from build123d import *

# Parameters (mm, degrees)
BOSS_EXTRUDE1_DEPTH = 2
SKETCH2_R           = 1.5
CUT_EXTRUDE1_DEPTH  = 31.987900865
SKETCH3_R           = 2.25
SKETCH3_R_2         = 1.5
BOSS_EXTRUDE2_DEPTH = 0.5
FILLET1_R           = 5


with BuildPart() as part:
    # Sketch1 → Boss-Extrude1 (new body)
    with BuildSketch(Plane(origin=(0, 0, 0), x_dir=(1, 0, 0), z_dir=(0, 1, 0))):
        with BuildLine():
            Line((7.5, 22.5), (7.5, -22.5))
            ThreePointArc((7.5, -22.5), (0, -30), (-7.5, -22.5))
            Line((-7.5, -22.5), (-7.5, 22.5))
            ThreePointArc((-7.5, 22.5), (0, 30), (7.5, 22.5))
        make_face()
    extrude(amount=BOSS_EXTRUDE1_DEPTH)

    # Sketch2 → Cut-Extrude1 (cut, through all)
    with BuildSketch(Plane(origin=(0, 2, 0), x_dir=(1, 0, 0), z_dir=(0, 1, 0))):
        with Locations(Location((0, 22.5, 0), (0, 0, 270))):
            Circle(SKETCH2_R)
        with Locations(Location((0, -22.5, 0), (0, 0, 270))):
            Circle(SKETCH2_R)
    extrude(amount=-CUT_EXTRUDE1_DEPTH, mode=Mode.SUBTRACT)

    # Sketch3 → Boss-Extrude2 (add)
    # profile 1 of 2: a face of its own
    with BuildSketch(Plane.XZ):
        with Locations(Location((0, 22.5, 0), (0, 0, 90))):
            Circle(SKETCH3_R)
        with Locations(Location((0, 22.5, 0), (0, 0, 90))):
            Circle(SKETCH3_R_2, mode=Mode.SUBTRACT)
    # profile 2 of 2: a face of its own
    with BuildSketch(Plane.XZ):
        with Locations(Location((0, -22.5, 0), (0, 0, 90))):
            Circle(SKETCH3_R)
        with Locations(Location((0, -22.5, 0), (0, 0, 90))):
            Circle(SKETCH3_R_2, mode=Mode.SUBTRACT)
    extrude(amount=BOSS_EXTRUDE2_DEPTH)

    # Fillet1
    # the kernel refuses this fillet: 5 mm, written as the material it adds along each edge
    with BuildSketch(Plane(origin=(0, 0, 22.5), x_dir=(0, 0, 1), z_dir=(1, 0, 0))) as fillet1_piece_1:
        with BuildLine():
            CenterArc((4.429449472, 5), FILLET1_R, 244.158067237, 25.841932763)
            Line((2.25, 0.5), (2.206411011, 0.41))
            ThreePointArc((2.206411011, 0.41), (2.15, 0.25), (2.15, 0))
            Line((2.15, 0), (2.25, -0.1))
            Line((2.25, -0.1), (4.429449472, -0.1))
            Line((4.429449472, -0.1), (4.429449472, 0))
        make_face()
    revolve(axis=Axis((0, 0, 22.5), (0, -1, 0)))
    with BuildSketch(Plane(origin=(0, 0, -22.5), x_dir=(0, 0, 1), z_dir=(1, 0, 0))) as fillet1_piece_2:
        with BuildLine():
            CenterArc((4.429449472, 5), FILLET1_R, 244.158067237, 25.841932763)
            Line((2.25, 0.5), (2.206411011, 0.41))
            ThreePointArc((2.206411011, 0.41), (2.15, 0.25), (2.15, 0))
            Line((2.15, 0), (2.25, -0.1))
            Line((2.25, -0.1), (4.429449472, -0.1))
            Line((4.429449472, -0.1), (4.429449472, 0))
        make_face()
    revolve(axis=Axis((0, 0, -22.5), (0, -1, 0)))


solid = part.part
Model file for the job. Use its own axes, mm. Coordinates: 2 decimals unless noted, no trailing zeros. Order: outer loops, then holes, each group sorted by start corner. A loop starts at its lowest first (then second) coordinate and runs counter-clockwise, first axis right, second up. Notation, with made-up numbers: (63, 8.25) -> (80, 8.25) arc R18 ccw to (80, 19.25) -> close; hole circle Ø6 at (0.5, 11.5). An arc over 180 degrees is marked (long way). Return JSON: item names as keys, results as strings. Group by question number.
Item 1: Flat gauge pin, fed straight in: P1, Ø4, axis at x = 0, z = 22.5, coming from the +Y side. Where does the tip first touch, or does it go through?
Item 2: Saw through at B-B on x = 0. State how many separate pieces and enclosed holes the cut face has, then the cut area to 3 significant figures.
Item 3: Saw through at C-C on z = 0.5. Write the cut outline in (x, y), then the cut area to 3 significant figures.
Item 4: Saw through at D-D on x = 6.75. Write the cut outline in (y, z), then the cut area to 3 significant figures.
Item 5: Wall check: line 1 along Z through (x, y) = (0, 0.8); line 2 along Z through (x, y) = (-1.25, 0.95); line 3 along X through (y, z) = (1.4, -22.5). Give the ranges that are in metal, low to high. Write a range as [from, to].
Item 6: Pull direction Z, two halves, no side cores. Call faces 1 (the cylindrical face through (0, 1, -24)), 2 (the cylindrical face through (0, 1, 30)), 3 (the cylindrical face through (0, 1, 21)), 4 (the flat face through (0, 2, 0)): pulls with the +Z half, pulls with the -Z half, needs draft (parallel to the pull), parting line crosses it, or undercut.
Item 7: Saw through at A-A on y = 0.55. Write the cut outline in (x, z), then the cut area to 3 significant figures.
Values found:
{
 "1": {"P1": "stops at y = 2"},
 "2": {"separate pieces": "3", "enclosed holes": "0", "area": "111 mm2"},
 "3": {"outline": "(-7.5, 0) -> (7.5, 0) -> (7.5, 2) -> (-7.5, 2) -> close", "area": "30.0 mm2"},
 "4": {"outline": "(0, -25.77) -> (2, -25.77) -> (2, 25.77) -> (0, 25.77) -> close", "area": "103 mm2"},
 "5": {"line 1": "z = [-30, -24], [-21, 21], [24, 30]", "line 2": "z = [-29.9, -23.33], [-21.67, 21.67], [23.33, 29.9]", "line 3": "x = [-7.5, -1.5], [1.5, 7.5]"},
 "6": {"face 1": "undercut", "face 2": "pulls with the +Z half", "face 3": "undercut", "face 4": "needs draft"},
 "7": {"outline": "(-7.5, -22.5) arc R7.5 ccw to (7.5, -22.5) -> (7.5, 22.5) arc R7.5 ccw to (-7.5, 22.5) -> close; hole circle Ø3 at (0, -22.5); hole circle Ø3 at (0, 22.5)", "area": "838 mm2"}
}
